Autodesk Inventor part; units mm, degrees
ref_plane "YZ Plane" through (0, 0, 0) normal (1, 0, 0) x (0, 1, 0)
ref_plane "XZ Plane" through (0, 0, 0) normal (0, 1, 0) x (-1, 0, 0)
ref_plane "XY Plane" through (0, 0, 0) normal (0, 0, 1) x (1, 0, 0)
sketch "Sketch1" plane through (0, 0, 0) normal (0, 1, 0) x (-1, 0, 0)
  line L0 (0, 0) -> (-20.32, 0)
  line L1 (-20.32, 0) -> (-20.32, -76.2)
  line L2 (-20.32, -76.2) -> (0, -76.2)
  line L3 (0, -76.2) -> (0, 0)
  dimension "d0" = 20.32
  dimension "d1" = 76.2
extrude "Extrusion1" add sketch "Sketch1" along normal blind 7.62
sketch "Sketch2" plane through (0, 7.62, 0) normal (0, 1, 0) x (1, 0, 0)
  line L0 (0, 0) -> (0, 12.7)
  line L1 (0, 12.7) -> (20.32, 12.7)
  line L2 (20.32, 12.7) -> (20.32, 63.5)
  line L3 (20.32, 63.5) -> (0, 63.5)
  line L4 (0, 63.5) -> (0, 12.7)
  dimension "d4" = 12.7
  dimension "d5" = 20.32
  dimension "d6" = 50.8
extrude "Extrusion2" add sketch "Sketch2" along normal blind 43.18
sketch "Sketch3" plane through (20.32, 0, 0) normal (1, 0, 0) x (0, 0, -1)
  line L0 (12.7, 50.8) -> (63.5, 50.8)
  line L1 (38.1, 50.8) -> (38.1, 25.4)
  circle A0 centre (38.1, 25.4) radius 19.05
  point P0 (0, 0)
  dimension "d9" = 25.4
  dimension "d10" = 38.1
extrude "Extrusion3" cut sketch "Sketch3" against normal blind 15.24
fillet "Fillet1" radius 25.4 2 edges at (10.16, 50.8, -63.5) (10.16, 50.8, -12.7)
sketch "Sketch6" plane through (0, 7.62, 0) normal (0, 1, 0) x (1, 0, 0)
  line L0 (0, 0) -> (20.32, 0)
  line L1 (10.16, 0) -> (10.16, 6.35)
  line L2 (20.32, 76.2) -> (0, 76.2)
  line L3 (10.16, 76.2) -> (10.16, 69.85)
  dimension "d20" = 6.35
  dimension "d21" = 6.35
fillet "Fillet2" radius 25.4 2 edges at (10.16, 7.62, -63.5) (10.16, 7.62, -12.7)
hole "Hole1" at (10.16, 7.62, -6.35) at (10.16, 7.62, -69.85) direction (0, -1, 0) diameter 5.08 end through all counterbore diameter 10.16 counterbore depth 3.81
sketch "Sketch7" plane through (10.16, 7.62, -6.35) normal (0, -1, 0) x (1, 0, 0)
  circle A0 centre (0, 0) radius 5.08
  circle A1 centre (0, -63.5) radius 2.54
  line L0 (-2.54, -63.5) -> (0, -63.5)
  circle A2 centre (0, -63.5) radius 5.08
  point P0 (-10.16, 6.35)
  dimension "d30" = 10.16
  dimension "d31" = 10.16
extrude "Extrusion5" cut sketch "Sketch7" against normal blind 15.24 contours A0 | A1 | A2
sketch "Sketch10" plane through (5.08, 25.4, -38.1) normal (1, 0, 0) x (0, 0, -1)
  line L0 (0, 0) -> (0, 6.35)
  circle A0 centre (0, 6.35) radius 6.35
  point P0 (-38.1, -25.4)
  dimension "d65" = 6.35
extrude "Extrusion8" cut sketch "Sketch10" against normal blind 25.4
sketch "Sketch12" plane through (5.08, 25.4, -38.1) normal (1, 0, 0) x (0, 0, -1)
  circle A0 centre (0, 6.35) radius 6.35
  line L0 (0, 0) -> (14.3694, 0) construction
  line L1 (0, 0) -> (14.3694, 0) construction
  line L2 (0, 0) -> (-7.747, 13.4182)
  line L3 (0, 0) -> (15.494, 0) construction
  line L4 (0, 0) -> (7.747, 13.4182)
  line L5 (0, 0) -> (15.494, 0) construction
  circle A1 centre (-7.747, 13.4182) radius 1.651
  circle A2 centre (7.747, 13.4182) radius 1.651
  point P0 (-38.1, -25.4)
  dimension "d79" = 15.494
  dimension "d80" = 120
  dimension "d81" = 15.494
  dimension "d82" = 60
  dimension "d83" = 3.302
  dimension "d84" = 3.302
extrude "Extrusion9" cut sketch "Sketch12" against normal blind 25.4 contours A1 | A2
sketch "Sketch13" plane through (5.08, 25.4, -38.1) normal (1, 0, 0) x (0, 0, -1)
  circle A0 centre (0, 6.35) radius 6.35
  point P0 (-38.1, -25.4)
  point P1 (0, 0)
pattern_circular "Circular Pattern3" count 6 over 360 about axis through (5.08, 25.4, -38.1) along (1, 0, 0) of "Extrusion8", "Extrusion9"
properties part number "Motor Mount V2"
Here's how the part is built. I have some questions about the finished solid (model axes, mm). A direction names the side the tool comes from. Coordinates: 2 decimals unless noted, no trailing zeros. Order: outer loops, then holes, each group sorted by start corner. A loop starts at its lowest first (then second) coordinate and runs counter-clockwise, first axis right, second up. Notation, with made-up numbers: M 36,22.5 L 58,22.5 A23 ccw 58,43.5 Z; hole C 9.5,3 d9. An arc over 180 degrees is marked long. Answer as a JSON object with one key per item and string values. Group by question number.
(1) Which directions (+Z, -Z, +X, -X, +Y, -Y) give clear straight access to the entire face, cutting with the end or side of a thin tool? Please do faces 5 (the face through (2.6, 12.7, -38)), 6 (the face through (5.08, 34, -29)), 7 (the face through (11.74, 10.47, -65.02)).
(2) Suppose I cut it at B-B, the plane z = -69.85. Please give me the cut outline in (x, y), then the cut area to 3 significant figures.
(3) For pin 1 (5 mm diameter, centred on x = 8, z = -7.5, fed in from +Y); pin 2 (6 mm diameter, centred on x = 4, z = -57.5, fed in from -Y); pin 3 (3 mm diameter, centred on x = 15, y = 45, fed in from -Z); pin 4 (4 mm diameter, centred on y = 38.82, z = -45.85, fed in from +X), each with a flat end and sliding along its axis, tell me the tip position at first contact or that it passes through.
(4) Suppose I cut it at D-D, the plane y = 43. Please give me the cut outline in (x, z), then the cut area to 3 significant figures.
(5) Suppose I cut it at A-A, the plane x = 11. State how many separate pieces and enclosed holes the cut face has, then the cut area to 3 significant figures.
(6) If we mould it in two halves opening along Y, with no side actions, what happens to faces 1 (the face through (10.02, 44.29, -55.08)), 2 (the face through (2.58, 18.97, -49.05)), 3 (the face through (10, 0, -38)), 4 (the face through (2.576, 12.986, -47.157))? For each: released by +Y, released by -Y, zero draft, split by the parting line, or undercut.
(7) I need wall thicknesses on probe 1 along Y at (x, z) = (9.25, -38.1); probe 2 along Z at (x, y) = (13.5, 8.5); probe 3 along Z at (x, y) = (17.5, 18.5). Which ranges of each line are inside material? Lowest first, please.
Values found:
{
 "1": {"face 5": "+X, -X", "face 6": "+X", "face 7": "+Y"},
 "2": {"outline": "M 0,0 L 7.62,0 L 7.62,3.81 L 5.08,3.81 L 5.08,12.72 L 0,12.72 Z; M 12.7,0 L 20.32,0 L 20.32,12.72 L 15.24,12.72 L 15.24,3.81 L 12.7,3.81 Z", "area": "149 mm^2"},
 "3": {"pin 1": "stops at y = 3.81", "pin 2": "stops at y = 0", "pin 3": "stops at z = -55.92", "pin 4": "stops at x = 5.08"},
 "4": {"outline": "M 0,-56.41 L 20.32,-56.41 L 20.32,-45.39 L 5.08,-45.39 L 5.08,-30.81 L 20.32,-30.81 L 20.32,-19.79 L 0,-19.79 Z", "area": "522 mm^2"},
 "5": {"separate pieces": "3", "enclosed holes": "1", "area": "1,290 mm^2"},
 "6": {"face 1": "released by +Y", "face 2": "undercut", "face 3": "released by -Y", "face 4": "undercut"},
 "7": {"probe 1": "y = 0 to 6.35, 44.45 to 50.8", "probe 2": "z = -74.76 to -73.68, -66.02 to -46.89, -29.31 to -10.18, -2.52 to -1.44", "probe 3": "z = -65.93 to -55.86, -20.34 to -10.27"}
}
